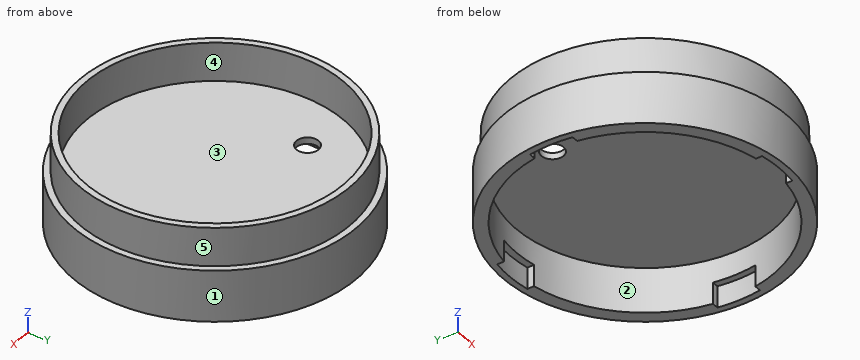
from build123d import *

# Parameters (mm, degrees)
F3_DEPTH = 5
F4_R     = 2.58
F5_DEPTH = 25


# Not quite as in the source:
# - ends of sketch curves that miss each other by under 0.0002 mm in the source are joined


with BuildPart() as f1:
    # F0 (on Front) → F1 (revolve)
    with BuildSketch(Plane.XZ):
        Polygon((30, 0), (0, 0), (0, -1.5), (30, -1.5), (30, -12), (33, -12), (33, 0), (31.5, 0), (31.5, 9), (30, 9), align=None)
    revolve(axis=Axis((0, 0, -0.75), (0, 0, 1)))

    # F2 (on face) → F3 (cut)
    with BuildSketch(Plane(origin=(0, 0, -12), x_dir=(1, 0, 0), z_dir=(0, 0, -1))):
        with BuildLine():
            Line((-5, 31.030934304), (-5, 29.5803989155))
            ThreePointArc((-5, 29.5803989155), (0, 30), (5, 29.5803989155))
            Line((5, 29.5803989155), (5, 31.0276464719))
            ThreePointArc((5, 31.0276464719), (0.0001313019, 31.4286473296), (-5, 31.030934304))
        make_face()
        with BuildLine():
            Line((-29.5821256825, 4.9897735526), (-31.1022785476, 4.9897735526))
            ThreePointArc((-31.1022785476, 4.9897735526), (-31.5, 0), (-31.1022852718, -4.9897746313))
            Line((-31.1022852718, -4.9897746313), (-29.5821255005, -4.9897746313))
            ThreePointArc((-29.5821255005, -4.9897746313), (-30, -5.47e-07), (-29.5821256825, 4.9897735526))
        make_face()
        with BuildLine():
            ThreePointArc((5, -29.5803989155), (0, -30), (-5, -29.5803989155))
            Line((-5, -29.5803989155), (-5, -31.1736362396))
            ThreePointArc((-5, -31.1736362396), (0.0001313019, -31.5713492653), (5, -31.1703484075))
            Line((5, -31.1703484075), (5, -29.5803989155))
        make_face()
        with BuildLine():
            Line((31.1022785476, 4.9897735526), (29.5821256825, 4.9897735526))
            ThreePointArc((29.5821256825, 4.9897735526), (29.8953488897, 2.5036203312), (30, 0))
            ThreePointArc((30, 0), (29.8953488441, -2.5036208763), (29.5821255005, -4.9897746313))
            Line((29.5821255005, -4.9897746313), (31.1022852718, -4.9897746313))
            ThreePointArc((31.1022852718, -4.9897746313), (31.5, 0), (31.1022785476, 4.9897735526))
        make_face()
    extrude(amount=-F3_DEPTH, mode=Mode.SUBTRACT)

    # F4 (on face) → F5 (cut)
    with BuildSketch(Plane.XY.offset(9)):
        with Locations((-17.3232257366, 9.4686336815)):
            Circle(F4_R)
    extrude(amount=-F5_DEPTH, mode=Mode.SUBTRACT)


solid = f1.part
Read the model definition and answer for the solid it produces. Units are mm, in the model's axes. Face numbers are marked on the shaded views. A direction names the side the tool comes from. Give positions to 0.01 mm unless a question says otherwise; leave off trailing zeros. Write each loop counter-clockwise with the first axis right and the second up, starting at its lowest first coordinate (ties: lowest second). Pieces come first, ordered by that corner, then holes. Notation, with made-up numbers: M -1.75,-24.5 L 3.25,-24.5 A25 cw 3.25,-9.5 Z; hole C 39.5,51 d10. An arc over 180 degrees is marked long. One line per item, written item: value. Start each with the question number.
(1) Find section B-B (x = 0). Determine the outline of the cut face in (y, z).
(2) A tool of negligible diameter and unlimited length cuts with its end or side. For the marked faces 1, 2 and 3, from which of +Z, -Z, +X, -X, +Y, -Y can it reach the whole face along a straight path? Write none if from no direction.
(3) Determine the mould class of the marked faces 4 and 5 for opening direction X: pulls with the +X half, pulls with the -X half, needs draft (parallel to the pull), parting line crosses it, or undercut.
(4) Find section A-A (z = -8.75). Determine the outline of the cut face in (x, y), plus the area to 3 significant figures.
(5) Find the intervals of material crossed by line 1 (Y direction, x = 0, z = -8.25); line 2 (Z direction, x = -4.5, y = 7.5); line 3 (X direction, y = -6, z = 2.5), in increasing order.
(6) Flat-ended cylindrical pins translate along their axes: pin 1 Ø0.6 at (x, y) = (30.5, -1.5) entering from -Z; pin 2 Ø1.2 at (x, z) = (-30, -9) entering from -Y; pin 3 Ø12 at (x, y) = (-10, -5) entering from +Z; pin 4 Ø10 at (x, y) = (-13, 23) entering from -Z. Find the tip coordinate at first contact, or state that the pin passes through.
(7) Find section D-D (x = 13). Determine the outline of the cut face in (y, z).
(8) Find section C-C (y = 0). Determine the outline of the cut face in (x, z).
Results below:
1. outline: M -33,-12 L -31.43,-12 L -31.43,-7 L -30,-7 L -30,-1.5 L 30,-1.5 L 30,-7 L 31.57,-7 L 31.57,-12 L 33,-12 L 33,0 L 31.5,0 L 31.5,9 L 30,9 L 30,0 L -30,0 L -30,9 L -31.5,9 L -31.5,0 L -33,0 Z
2. face 1: +Z, -Z
2. face 2: -Z
2. face 3: +Z
3. face 4: undercut
3. face 5: parting line crosses it
4. outline: C 0,0 d66; hole M -31.1,-4.99 L -29.58,-4.99 A30 ccw -5,-29.58 L -5,-31.03 A31.5 ccw 5,-31.03 L 5,-29.58 A30 ccw 29.58,-4.99 L 31.1,-4.99 A31.5 ccw 31.1,4.99 L 29.58,4.99 A30 ccw 5,29.58 L 5,31.17 A31.5 ccw -5,31.17 L -5,29.58 A30 ccw -29.58,4.99 L -31.1,4.99 A31.5 ccw Z
4. area: 534 mm^2
5. line 1: y = -33 to -31.43, 31.57 to 33
5. line 2: z = -1.5 to 0
5. line 3: x = -30.92 to -29.39, 29.39 to 30.92
6. pin 1: stops at z = -7
6. pin 2: stops at y = -14.99
6. pin 3: stops at z = 0
6. pin 4: stops at z = -12
7. outline: M -30.33,-12 L -27.04,-12 L -27.04,-1.5 L 27.04,-1.5 L 27.04,-12 L 30.33,-12 L 30.33,0 L 28.69,0 L 28.69,9 L 27.04,9 L 27.04,0 L -27.04,0 L -27.04,9 L -28.69,9 L -28.69,0 L -30.33,0 Z
8. outline: M -33,-12 L -31.5,-12 L -31.5,-7 L -30,-7 L -30,-1.5 L 30,-1.5 L 30,-7 L 31.5,-7 L 31.5,-12 L 33,-12 L 33,0 L 31.5,0 L 31.5,9 L 30,9 L 30,0 L -30,0 L -30,9 L -31.5,9 L -31.5,0 L -33,0 Z
